```python
from build123d import *

# Parameters (mm, degrees)
SKETCH1_W                      = 571.5
SKETCH1_H                      = 571.5
PLATE_DEPTH                    = 15
SKETCH2_R                      = 87.5
BEARING_HOLE_DEPTH             = 405.389818121
CBORE_FOR_M10_SHCS_D           = 12
CBORE_FOR_M10_SHCS_CBORE_D     = 18
CBORE_FOR_M10_SHCS_CBORE_DEPTH = 10
SKETCH7_W                      = 546
SKETCH7_H                      = 546
SKETCH7_W_2                    = 540
SKETCH7_H_2                    = 540
CUT_EXTRUDE1_DEPTH             = 5


with BuildPart() as part:
    # Sketch1 → plate (new body)
    with BuildSketch(Plane(origin=(0, 0, 0), x_dir=(1, 0, 0), z_dir=(0, 1, 0))):
        Rectangle(SKETCH1_W, SKETCH1_H)
    extrude(amount=PLATE_DEPTH)

    # Sketch2 → bearing-hole (cut, through all)
    with BuildSketch(Plane(origin=(0, 15, 0), x_dir=(1, 0, 0), z_dir=(0, 1, 0))):
        with Locations(Location((0, 0, 0), (0, 0, 270))):
            Circle(SKETCH2_R)
    extrude(amount=-BEARING_HOLE_DEPTH, mode=Mode.SUBTRACT)

    # CBORE for M10 SHCS (through all)
    with Locations(Plane(origin=(0, 15, 0), x_dir=(1, 0, 0), z_dir=(0, 1, 0))):
        with Locations((0, 0), (-106.066017178, 0), (0, 106.066017178), (106.066017178, 0), (0, -106.066017178), (176.776695297, 176.776695297), (-176.776695297, 176.776695297), (176.776695297, -176.776695297), (-176.776695297, -176.776695297)):
            CounterBoreHole(CBORE_FOR_M10_SHCS_D / 2, CBORE_FOR_M10_SHCS_CBORE_D / 2, CBORE_FOR_M10_SHCS_CBORE_DEPTH)

    # Sketch7 → Cut-Extrude1 (cut)
    with BuildSketch(Plane(origin=(0, 15, 0), x_dir=(1, 0, 0), z_dir=(0, 1, 0))):
        Rectangle(SKETCH7_W, SKETCH7_H)
        Rectangle(SKETCH7_W_2, SKETCH7_H_2, mode=Mode.SUBTRACT)
    extrude(amount=-CUT_EXTRUDE1_DEPTH, mode=Mode.SUBTRACT)


solid = part.part
```
Verification items for the finished model (mm, model axes). A direction names the side the tool comes from. Round coordinates to 2 decimals unless told otherwise and drop trailing zeros. Write each loop counter-clockwise with the first axis right and the second up, starting at its lowest first coordinate (ties: lowest second). Pieces come first, ordered by that corner, then holes. Notation, with made-up numbers: (8.5, 12) -> (58.5, 12) arc R28 cw to (58.5, 38) -> close; hole circle Ø9 at (38, -16). An arc over 180 degrees is marked (long way). Write each question's results on one line, items separated by ' | '. Start each with the question number.
1. Cross-section at B-B (x = 49.5). Enter the section's corners in (y, z), then the cut area to 3 significant figures.
2. Set-up check for faces 5 (the cylindrical face through (86.755, 7.605, -11.391)), 6 (the cylindrical face through (-1.95, 10.07, -97.28)): record each of +Z, -Z, +X, -X, +Y, -Y from which the full face is reachable in a straight line by a thin tool's end or side.
3. Material ranges on probe 1 along X at (y, z) = (13.5, -186); probe 2 along Z at (x, y) = (175, 1.25), recorded low to high. Write a range as from..to.
4. Depth check by flat-ended pin: P1, Ø9, axis at x = -103, z = -1.5, coming from the +Y side. Enter the tip coordinate at first touch or a pass-through.
5. Draft check along X on faces 1 (the flat face through (-285.75, 7, 4)), 2 (the flat face through (285.75, 7, 4)), 3 (the cylindrical face through (-97.48, 10.07, -2.7)), 4 (the cylindrical face through (-168.463, 10.07, -173.33)). Enter one of: +X half, -X half, draft (parallel to the pull), parting line (faces both ways), or undercut.
6. Cross-section at A-A (z = 58). Enter the section's corners in (x, y), then the cut area to 3 significant figures.
7. Cross-section at C-C (y = 7.75). Count the separate pieces of the cut face and the enclosed holes in it, then the cut area to 3 significant figures.
Solutions:
1) outline: (0, -285.75) -> (15, -285.75) -> (15, -273) -> (10, -273) -> (10, -270) -> (15, -270) -> (15, -72.15) -> (0, -72.15) -> close; (0, 72.15) -> (15, 72.15) -> (15, 270) -> (10, 270) -> (10, 273) -> (15, 273) -> (15, 285.75) -> (0, 285.75) -> close | area: 6,380 mm2
2) face 5: +Y, -Y | face 6: +Y
3) probe 1: x = -285.75..-273, -270..270, 273..285.75 | probe 2: z = -285.75..-182.51, -171.05..171.05, 182.51..285.75
4) P1: stops at y = 5
5) face 1: -X half | face 2: +X half | face 3: undercut | face 4: undercut
6) outline: (-285.75, 0) -> (-65.52, 0) -> (-65.52, 15) -> (-270, 15) -> (-270, 10) -> (-273, 10) -> (-273, 15) -> (-285.75, 15) -> close; (65.52, 0) -> (285.75, 0) -> (285.75, 15) -> (273, 15) -> (273, 10) -> (270, 10) -> (270, 15) -> (65.52, 15) -> close | area: 6,580 mm2
7) separate pieces: 1 | enclosed holes: 9 | area: 301,000 mm2
